from build123d import *

# Parameters (mm, degrees)
SKETCH1_R           = 5
SKETCH1_R_2         = 1.25
BOSS_EXTRUDE1_DEPTH = 3
SKETCH2_W           = 28
SKETCH2_H           = 3
BOSS_EXTRUDE2_DEPTH = 33
FILLET1_R           = 1
SKETCH4_R           = 2
SKETCH4_R_2         = 5
CUT_EXTRUDE1_DEPTH  = 10


with BuildPart() as part:
    # Sketch1 → Boss-Extrude1 (new body)
    with BuildSketch(Plane.XY):
        with BuildLine():
            Line((-14, 0), (-14, -19))
            Line((-14, -19), (14, -19))
            Line((14, -19), (14, 0))
            ThreePointArc((14, 0), (0, 14), (-14, 0))
        make_face()
        Circle(SKETCH1_R, mode=Mode.SUBTRACT)
        with Locations((-8.5, 0)):
            Circle(SKETCH1_R_2, mode=Mode.SUBTRACT)
        with Locations((8.5, 0)):
            Circle(SKETCH1_R_2, mode=Mode.SUBTRACT)
    extrude(amount=BOSS_EXTRUDE1_DEPTH)

    # Sketch2 → Boss-Extrude2 (add)
    with BuildSketch(Plane.XY.offset(3)):
        with Locations((0, -17.5)):
            Rectangle(SKETCH2_W, SKETCH2_H)
    extrude(amount=BOSS_EXTRUDE2_DEPTH)

    # Fillet1
    fillet1_edges = [part.edges().sort_by_distance(p)[0] for p in [
        (-14, -17.5, 36),
        (14, -17.5, 36),
        (0, -19, 0),
    ]]
    fillet(fillet1_edges, radius=FILLET1_R)

    # Sketch4 → Cut-Extrude1 (cut)
    with BuildSketch(Plane.XZ.offset(19)):
        with Locations((-9, 28)):
            Circle(SKETCH4_R)
        with Locations((-9, 13)):
            Circle(SKETCH4_R)
        with Locations((9, 28)):
            Circle(SKETCH4_R)
        with Locations((9, 13)):
            Circle(SKETCH4_R)
        with Locations((0, 20.5)):
            Circle(SKETCH4_R_2)
    extrude(amount=-CUT_EXTRUDE1_DEPTH, mode=Mode.SUBTRACT)


solid = part.part
Input: part model. Units: mm. Frame: model coordinates. A direction names the side the tool comes from. Coordinates: 2 decimals unless noted, no trailing zeros. Order: outer loops, then holes, each group sorted by start corner. A loop starts at its lowest first (then second) coordinate and runs counter-clockwise, first axis right, second up.
1. Cut plane D-D, the plane y = -0.5. Return loops of the section in (x, z).
Checked values:
outline: (-14, 0) - (-9.65, 0) - (-9.65, 3) - (-14, 3) - close; (-7.35, 0) - (-4.97, 0) - (-4.97, 3) - (-7.35, 3) - close; (4.97, 0) - (7.35, 0) - (7.35, 3) - (4.97, 3) - close; (9.65, 0) - (14, 0) - (14, 3) - (9.65, 3) - close
2. Draft query along X for faces 1 (the cylindrical face through (7.526, -17.521, 14.352)), 2 (the cylindrical face through (9, -18, 26)), 3 (the flat face through (0, -17, 36)), 4 (the flat face through (-14, -17, 14)). Return one class per face: +X half, -X half, draft (parallel to the pull), parting line (faces both ways), or undercut.
Checked values:
face 1: undercut
face 2: undercut
face 3: draft
face 4: -X half
3. Access query for faces 5 (the flat face through (-3.3, -4.1, 3)), 6 (the cylindrical face through (-9, -18, 15)). Directions: +Z, -Z, +X, -X, +Y, -Y. A direction counts if a zero-diameter tool reaches every point of the face in a straight line with its end or side. Return the directions, or none.
Checked values:
face 5: +Z, +X, -X, +Y
face 6: +Y, -Y
4. Ray query, line 1 along Z through (x, y) = (-9, -17.55); line 2 along Z through (x, y) = (0, -17.6); line 3 along Y through (x, z) = (-9.5, 31.5). Return the intervals inside material, ascending.
Checked values:
line 1: z = 0 to 11, 15 to 26, 30 to 36
line 2: z = 0 to 15.5, 25.5 to 36
line 3: y = -19 to -16
5. Cut plane A-A, the plane z = 20.5. Return loops of the section in (x, y), plus the area to 3 significant figures.
Checked values:
outline: (-14, -19) - (-5, -19) - (-5, -16) - (-14, -16) - close; (5, -19) - (14, -19) - (14, -16) - (5, -16) - close
area: 54.0 mm2
6. Contact query for flat-ended pins moving along their axis: P1, Ø4, axis at x = -11, y = -10.5, coming from the +Z side; P2, Ø5, axis at x = 9, z = 28, coming from the +Y side; P3, Ø6, axis at x = 0, y = 0, coming from the +Z side. Output: stop coordinate, or through.
Checked values:
P1: stops at z = 3
P2: stops at y = -16
P3: passes through
7. Cut plane B-B, the plane x = 0. Return loops of the section in (y, z), plus the area to 3 significant figures.
Checked values:
outline: (-19, 1) arc R1 ccw to (-18, 0) - (-5, 0) - (-5, 3) - (-16, 3) - (-16, 15.5) - (-19, 15.5) - close; (-19, 25.5) - (-16, 25.5) - (-16, 36) - (-19, 36) - close; (5, 0) - (14, 0) - (14, 3) - (5, 3) - close
area: 138 mm2
8. Cut plane C-C, the plane z = 13. Return loops of the section in (x, y).
Checked values:
outline: (-14, -19) - (-11, -19) - (-11, -16) - (-14, -16) - close; (-7, -19) - (7, -19) - (7, -16) - (-7, -16) - close; (11, -19) - (14, -19) - (14, -16) - (11, -16) - close
